Input: part model. Units: mm. Frame: model coordinates. Face numbers are marked on the shaded views. Coordinates: 2 decimals unless noted, no trailing zeros. Order: outer loops, then holes, each group sorted by start corner. A loop starts at its lowest first (then second) coordinate and runs counter-clockwise, first axis right, second up. Notation, with made-up numbers: (40, -19.5) -> (69, -19.5) arc R9 cw to (69, -9.5) -> close; hole circle Ø3 at (-35.5, -31). An arc over 180 degrees is marked (long way). Use CSV: the item, a comma, the result in double quotes. Start each with the question number.
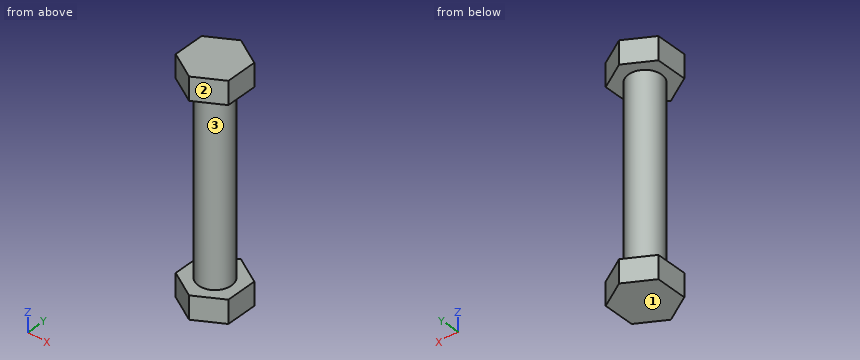
```python
from build123d import *

# Parameters (mm, degrees)
EXTRUDE_START      = -33
EXTRUDE_SKETCH_1_R = 5
EXTRUDE_1_DEPTH    = 66
EXTRUDE_START_2    = 28
EXTRUDE_2_DEPTH    = 7
EXTRUDE_START_3    = -35
EXTRUDE_3_DEPTH    = 7


with BuildPart() as part:
    # Extrude sketch 1 → Extrude 1 (new body)
    with BuildSketch(Plane.XY.offset(EXTRUDE_START)):
        Circle(EXTRUDE_SKETCH_1_R)
    extrude(amount=EXTRUDE_1_DEPTH)


with BuildPart() as body_2:
    # Extrude sketch 2 → Extrude 2 (new body)
    with BuildSketch(Plane.XY.offset(EXTRUDE_START_2)):
        Polygon((8, 4.618802154), (0, 9.237604307), (-8, 4.618802154), (-8, -4.618802154), (0, -9.237604307), (8, -4.618802154), align=None)
    extrude(amount=EXTRUDE_2_DEPTH)


with BuildPart() as body_3:
    # Extrude sketch 3 → Extrude 3 (new body)
    with BuildSketch(Plane.XY.offset(EXTRUDE_START_3)):
        Polygon((8, 4.618802154), (0, 9.237604307), (-8, 4.618802154), (-8, -4.618802154), (0, -9.237604307), (8, -4.618802154), align=None)
    extrude(amount=EXTRUDE_3_DEPTH)

    # Combine (weld / assembly of features): union body 2, part
    add(body_2.part)
    add(part.part)


solid = body_3.part
```
1. Section A-A on x = 7.25. Return loops of the section in (y, z).
2. Material intervals for line 1 along Z through (x, y) = (5.5, -0.75); line 2 along X through (y, z) = (0, 5.5); line 3 along Y through (x, z) = (-1.75, -2.5), sorted ascending.
3. Section B-B on y = 0. Return loops of the section in (x, z).
4. Section C-C on y = -6. Return loops of the section in (x, z).
5. Contact query for flat-ended pins moving along their axis: P1, Ø1.5, axis at x = -4, z = -26.5, coming from the +Y side; P2, Ø5, axis at x = 3, z = -13, coming from the +Y side; P3, Ø1.5, axis at x = -2, z = 1, coming from the +Y side. Output: stop coordinate, or through.
6. Pull-direction query (Z, two-part tool) for the marked faces 1, 2 and 3; classes: released by +Z, released by -Z, zero draft, split by the parting line, or undercut.
7. Section D-D on x = -1.5. Return loops of the section in (y, z).
Values follow:
1,outline,"(-5.05, -35) -> (5.05, -35) -> (5.05, -28) -> (-5.05, -28) -> close; (-5.05, 28) -> (5.05, 28) -> (5.05, 35) -> (-5.05, 35) -> close"
2,line 1,"z = -35 to -28, 28 to 35"
2,line 2,"x = -5 to 5"
2,line 3,"y = -4.68 to 4.68"
3,outline,"(-8, -35) -> (8, -35) -> (8, -28) -> (5, -28) -> (5, 28) -> (8, 28) -> (8, 35) -> (-8, 35) -> (-8, 28) -> (-5, 28) -> (-5, -28) -> (-8, -28) -> close"
4,outline,"(-5.61, -35) -> (5.61, -35) -> (5.61, -28) -> (-5.61, -28) -> close; (-5.61, 28) -> (5.61, 28) -> (5.61, 35) -> (-5.61, 35) -> close"
5,P1,"stops at y = 3.8"
5,P2,"stops at y = 4.97"
5,P3,"stops at y = 4.84"
6,face 1,"released by -Z"
6,face 2,"zero draft"
6,face 3,"undercut"
7,outline,"(-8.37, -35) -> (8.37, -35) -> (8.37, -28) -> (4.77, -28) -> (4.77, 28) -> (8.37, 28) -> (8.37, 35) -> (-8.37, 35) -> (-8.37, 28) -> (-4.77, 28) -> (-4.77, -28) -> (-8.37, -28) -> close"
